Autodesk Inventor part; units mm, degrees
ref_plane "YZ Plane" through (0, 0, 0) normal (1, 0, 0) x (0, 1, 0)
ref_plane "XZ Plane" through (0, 0, 0) normal (0, 1, 0) x (-1, 0, 0)
ref_plane "XY Plane" through (0, 0, 0) normal (0, 0, 1) x (1, 0, 0)
ref_plane "Work Plane5" through (0, 0, 10) normal (0, 0, 1) x (1, 0, 0)
sketch "Sketch1" plane through (0, 0, 10) normal (0, 0, 1) x (1, 0, 0)
  line L0 (-4.0299, -0.3538) -> (-2.2322, 1.4439) construction
  arc A0 (-1.4439, 2.2322) -> (-2.2322, 1.4439) centre (-0.9299, 0.9299) ccw construction
  line L1 (-1.4439, 2.2322) -> (0.3538, 4.0299) construction
  line L2 (-37.8299, 42.8299) -> (-37.8299, 37.8299) construction
  line L3 (-37.8299, 37.8299) -> (-42.9208, 37.8299) construction
  line L4 (-37.8299, 42.2137) -> (-37.8299, 45.8299) construction
  line L5 (-37.8299, 45.8299) -> (-4.0299, 45.8299) construction
  line L6 (-4.0299, 45.8299) -> (-4.0299, 42.2137) construction
  line L7 (-4.0299, 4.0299) -> (0.3538, 4.0299)
  circle A1 centre (-20.9299, 20.9299) radius 17.5
  line L8 (-20.9299, 58.9723) -> (17.1124, 20.9299) construction
  line L9 (17.1124, 20.9299) -> (-20.9299, -17.1124) construction
  line L10 (-20.9299, -17.1124) -> (-58.9723, 20.9299) construction
  line L11 (-58.9723, 20.9299) -> (-20.9299, 58.9723) construction
  line L12 (-20.9299, 58.9723) -> (-20.9299, -17.1124) construction
  line L13 (17.1124, 20.9299) -> (-58.9723, 20.9299) construction
  line L14 (-20.9299, 58.9723) -> (32.8701, 58.9723) construction
  line L15 (-43.4299, 43.4299) -> (1.5701, 43.4299) construction
  line L16 (1.5701, 43.4299) -> (1.5701, -1.5701) construction
  line L17 (1.5701, -1.5701) -> (-43.4299, -1.5701) construction
  line L18 (-43.4299, -1.5701) -> (-43.4299, 43.4299) construction
  line L19 (-43.4299, 43.4299) -> (1.5701, -1.5701) construction
  line L20 (1.5701, 43.4299) -> (-43.4299, -1.5701) construction
  line L21 (-43.4299, 5.3876) -> (-43.4299, 36.4723)
  line L22 (-43.4299, 36.4723) -> (-36.4723, 43.4299)
  line L23 (-36.4723, 43.4299) -> (-5.3876, 43.4299)
  line L24 (-5.3876, 43.4299) -> (1.5701, 36.4723)
  line L25 (1.5701, 36.4723) -> (1.5701, 5.3876)
  line L26 (1.5701, 5.3876) -> (-5.3876, -1.5701)
  line L27 (-5.3876, -1.5701) -> (-36.4723, -1.5701)
  line L28 (-36.4723, -1.5701) -> (-43.4299, 5.3876)
  line L29 (-4.0299, 42.2137) -> (-37.8299, 42.2137)
  line L30 (-4.0299, -0.3538) -> (-4.0299, 4.0299)
  circle A2 centre (-20.9299, 20.9299) radius 1.5
  line L31 (-10.9299, 10.9299) -> (-30.9299, 10.9299) construction
  line L32 (-30.9299, 10.9299) -> (-30.9299, 30.9299) construction
  line L33 (-30.9299, 30.9299) -> (-10.9299, 30.9299) construction
  line L34 (-10.9299, 30.9299) -> (-10.9299, 10.9299) construction
  line L35 (-10.9299, 10.9299) -> (-30.9299, 30.9299) construction
  line L36 (-30.9299, 10.9299) -> (-10.9299, 30.9299) construction
  circle A3 centre (-30.9299, 30.9299) radius 1.4
  circle A4 centre (-30.9299, 10.9299) radius 1.4
  circle A5 centre (-10.9299, 10.9299) radius 1.4
  line L37 (-45.8299, 37.8299) -> (-42.0723, 37.8299) construction
  line L38 (-42.1723, 37.7299) -> (-45.8299, 37.7299)
  line L39 (-45.8299, 37.7299) -> (-45.8299, 4.1299)
  line L40 (-45.8299, 4.1299) -> (-42.1723, 4.1299)
  line L41 (-42.1723, 4.1299) -> (-42.1723, 37.7299)
  line L42 (-45.8299, 4.0299) -> (-42.0723, 4.0299) construction
  line L43 (-45.8299, 37.8299) -> (-42.0723, 37.8299)
  line L44 (-37.7299, 45.8299) -> (-4.1299, 45.8299)
  line L45 (-4.1299, 45.8299) -> (-4.1299, 42.1723)
  line L46 (-4.1299, 42.1723) -> (-37.7299, 42.1723)
  line L47 (-37.7299, 42.1723) -> (-37.7299, 45.8299)
  line L48 (0.4701, 37.8299) -> (0.4701, 4.0299) construction
  line L49 (0.4701, 4.0299) -> (3.9701, 4.0299) construction
  line L50 (3.9701, 37.8299) -> (3.9701, 4.0299) construction
  line L51 (0.4701, 37.8299) -> (3.9701, 37.8299) construction
  line L52 (-45.8299, -3.9701) -> (-4.0299, -3.9701) construction
  line L53 (0.3124, 37.7299) -> (3.9701, 37.7299)
  line L54 (3.9701, 37.7299) -> (3.9701, 4.1299)
  line L55 (3.9701, 4.1299) -> (0.3124, 4.1299)
  line L56 (0.3124, 4.1299) -> (0.3124, 37.7299)
  line L57 (-4.1713, -0.3538) -> (-37.7299, -0.3538)
  line L58 (-37.7299, -0.3538) -> (-37.7299, -3.9701)
  line L59 (-37.7299, -3.9701) -> (-4.1713, -3.9701)
  line L60 (-4.1713, -3.9701) -> (-4.1713, -0.3538)
  point P0 (-37.8299, 4.0299)
  dimension "d18" = 53.8
  dimension "d19" = 45
  dimension "d20" = 53.8
  dimension "d21" = 45
  dimension "d22" = 45
  dimension "d30" = 20
  dimension "d31" = 20
  dimension "d32" = 2.8
  dimension "d33" = 2.8
  dimension "d34" = 2.8
  dimension "d35" = 3
  dimension "d36" = 0.1
  dimension "d37" = 0.1
  dimension "d38" = 0.1
  dimension "d39" = 0.1
extrude "Extrusion1" add sketch "Sketch1" along normal blind 15 contours L30 L26 L57 L28 L41 L22 L46 L24 L56 L7 | L7 L26 L30 | L56 L24 L25 L26 | L26 L25 L24 L53 L54 L55 | L60 L59 L58 L57 L28 L27 L26 | L26 L27 L28 L57 | L46 L22 L29 L24 | L24 L29 L45 | L40 L39 L38 L22 L21 L28 | L28 L21 L22 L41 | L29 L22 L23 L24 | L24 L23 L22 L29 L47 L44 L45 | L47 L29 L22 | A1 | A2 | A3 | A4 | A5
sketch "Skizze4" plane through (0, 0, 25) normal (0, 0, 1) x (1, 0, 0)
  line L0 (-37.7299, 42.1723) -> (-42.1723, 37.7299)
  line L1 (-42.1723, 37.7299) -> (-45.8299, 37.7299)
  line L2 (-45.8299, 37.7299) -> (-45.8299, 4.1299) construction
  line L3 (-45.8299, 4.1299) -> (-42.1723, 4.1299)
  line L4 (-42.1723, 4.1299) -> (-37.6885, -0.3538)
  line L5 (-37.6885, -0.3538) -> (-37.7299, -0.3538)
  line L6 (-37.7299, -0.3538) -> (-37.7299, -3.9701)
  line L7 (-37.7299, -3.9701) -> (-4.1713, -3.9701) construction
  line L8 (-4.1713, -3.9701) -> (-4.1713, -0.3538)
  line L9 (-4.1713, -0.3538) -> (0.3124, 4.1299)
  line L10 (0.3124, 4.1299) -> (3.9701, 4.1299)
  line L11 (3.9701, 4.1299) -> (3.9701, 37.7299) construction
  line L12 (3.9701, 37.7299) -> (0.3124, 37.7299)
  line L13 (0.3124, 37.7299) -> (-4.1299, 42.1723)
  line L14 (-4.1299, 42.1723) -> (-4.1299, 45.8299)
  line L15 (-4.1299, 45.8299) -> (-37.7299, 45.8299) construction
  line L16 (-37.7299, 45.8299) -> (-37.7299, 42.1723)
  line L17 (-37.9299, 46.0299) -> (-3.9299, 46.0299) construction
  line L18 (-3.9299, 46.0299) -> (-3.9299, 42.2551)
  line L19 (-3.9299, 42.2551) -> (0.3953, 37.9299)
  line L20 (0.3953, 37.9299) -> (4.1701, 37.9299)
  line L21 (4.1701, 37.9299) -> (4.1701, 3.9299) construction
  line L22 (4.1701, 3.9299) -> (0.3953, 3.9299)
  line L23 (0.3953, 3.9299) -> (-3.9713, -0.4367)
  line L24 (-3.9713, -0.4367) -> (-3.9713, -4.1701)
  line L25 (-3.9713, -4.1701) -> (-37.9299, -4.1701) construction
  line L26 (-37.9299, -4.1701) -> (-37.9299, -0.3953)
  line L27 (-37.9299, -0.3953) -> (-42.2551, 3.9299)
  line L28 (-42.2551, 3.9299) -> (-46.0299, 3.9299)
  line L29 (-46.0299, 3.9299) -> (-46.0299, 37.9299) construction
  line L30 (-46.0299, 37.9299) -> (-42.2551, 37.9299)
  line L31 (-42.2551, 37.9299) -> (-37.9299, 42.2551)
  line L32 (-37.9299, 42.2551) -> (-37.9299, 46.0299)
  line L33 (-45.8299, 37.7299) -> (-45.8299, 37.9299)
  line L34 (-4.1299, 45.8299) -> (-37.7299, 45.8299)
  line L35 (-37.7299, 45.8299) -> (-37.9299, 45.8299)
  line L36 (-4.1299, 45.8299) -> (-3.9299, 45.8299)
  line L37 (3.9701, 37.7299) -> (3.9701, 37.9299)
  line L38 (3.9701, 4.1299) -> (3.9701, 37.7299)
  line L39 (3.9701, 4.1299) -> (3.9701, 3.9299)
  line L40 (-4.1713, -3.9701) -> (-3.9713, -3.9701)
  line L41 (-37.7299, -3.9701) -> (-37.9299, -3.9701)
  line L42 (-45.8299, 4.1299) -> (-45.8299, 3.9299)
  point P0 (0, 0)
  dimension "d40" = 0.2
extrude "IM_offset" add sketch "Skizze4" against normal up to surface (15 mm away)
sketch "Sketch29" plane through (0, 0, 10) normal (0, 0, -1) x (-1, 0, 0)
  arc A0 (6.7299, 9.4299) -> (9.4299, 6.7299) centre (9.4299, 9.4299) ccw
  line L0 (9.4299, 6.7299) -> (32.4299, 6.7299)
  arc A1 (32.4299, 6.7299) -> (35.1299, 9.4299) centre (32.4299, 9.4299) ccw
  line L1 (35.1299, 9.4299) -> (35.1299, 32.4299)
  arc A2 (35.1299, 32.4299) -> (32.4299, 35.1299) centre (32.4299, 32.4299) ccw
  line L2 (32.4299, 35.1299) -> (9.4299, 35.1299)
  arc A3 (9.4299, 35.1299) -> (6.7299, 32.4299) centre (9.4299, 32.4299) ccw
  line L3 (6.7299, 32.4299) -> (6.7299, 9.4299)
  line L4 (36.9299, 4.9299) -> (4.9299, 4.9299)
  line L5 (4.9299, 4.9299) -> (4.9299, 36.9299)
  line L6 (4.9299, 36.9299) -> (36.9299, 36.9299)
  line L7 (36.9299, 36.9299) -> (36.9299, 4.9299)
  line L8 (36.9299, 4.9299) -> (4.9299, 36.9299) construction
  line L9 (4.9299, 4.9299) -> (36.9299, 36.9299) construction
  point P0 (0, 0)
  point P1 (20.9299, 20.9299)
  dimension "d187" = 32
  dimension "d188" = 32
extrude "Extrusion23" cut sketch "Sketch29" against normal through all contours L3 A3 L2 A2 L1 A1 L0 A0 | L4 L5 L6 L7
sketch "Sketch30" plane through (-45.8299, 0, 10) normal (-1, 0, 0) x (0, 0, 1)
  line L0 (35.0799, 45.8299) -> (6.8799, 45.8299)
  line L1 (0, 3.9299) -> (0, 37.9299)
  line L2 (15, 3.9299) -> (0, 3.9299)
  line L3 (15, 37.9299) -> (15, 3.9299)
  line L4 (15, 37.9299) -> (0, 37.9299)
  circle A0 centre (7.5, 20.9299) radius 1.7201
  point P0 (-10, 0)
ref_plane "Arbeitsebene7" through (-20.9299, 3.9299, 10) normal (-1, 0, 0) x (0, 0, 1)
ref_plane "Arbeitsebene8" through (-37.9299, 20.9299, 10) normal (0, 1, 0) x (1, 0, 0)
ref_plane "Arbeitsebene9" through (-20.9299, 3.9299, 10) normal (-1, 0, 0) x (0, 0, 1)
ref_plane "Arbeitsebene10" through (-37.9299, 20.9299, 10) normal (0, -1, 0) x (1, 0, 0)
hole "Bohrung2" at (-45.8299, 20.9299, 17.5) direction (1, 0, 0) diameter 2.8 end through all counterbore diameter 6 counterbore depth 4
pattern_circular "Runde Anordnung2" count 4 over 360 about axis through (-20.9299, 20.9299, 10) along (0, 0, 1) of "Bohrung2"
ref_plane "Arbeitsebene11" through (-20.9299, 3.9299, 10) normal (1, 0, 0) x (0, 0, -1)
ref_plane "Arbeitsebene12" through (-37.9299, 20.9299, 10) normal (0, 1, 0) x (1, 0, 0)
properties part number "30_Cube_Z_Focus_MGN_NEMA_Motorsupport_centered"
CAD build for the part. Positions are in the model's coordinates, mm. A direction names the side the tool comes from. Round coordinates to 2 decimals unless told otherwise and drop trailing zeros. Order: outer loops, then holes, each group sorted by start corner. A loop starts at its lowest first (then second) coordinate and runs counter-clockwise, first axis right, second up. Notation, with made-up numbers: (2.25, 9) -> (21.25, 9) arc R16 cw to (21.25, 37) -> close; hole circle Ø10 at (-35.75, 43). An arc over 180 degrees is marked (long way). One line per question, with ' | ' between items.
Q1. Slice it at C-C (x = -3). Write the cut outline in (y, z), then the cut area to 3 significant figures.
Completed:
outline: (0.53, 10) -> (41.33, 10) -> (41.33, 25) -> (0.53, 25) -> close; hole circle Ø2.8 at (20.93, 17.5) | area: 606 mm^2
Q2. Which spindle directions (+Z, -Z, +X, -X, +Y, -Y) get a long thin tool onto all of the face, cutting with end or side? Do faces 4 (the flat face through (2, 3.93, 18)), 5 (the cylindrical face through (-43.802, 22.755, 15.119)), 6 (the flat face through (-37.93, -2, 18)). Say none if no direction does.
Completed:
face 4: +Z, -Z, +X, -Y | face 5: -X | face 6: +Z, -Z, -X, -Y
Q3. Two-plate mould, pull along Z, no slides. Class faces 1 (the flat face through (-22, 0.03, 19)), 2 (the flat face through (-4.93, 20.7, 15.7)), 3 (the flat face through (-21, 38, 10)): released by +Z, released by -Z, zero draft, split by the parting line, or undercut.
Completed:
face 1: undercut | face 2: zero draft | face 3: released by -Z
Q4. Probe probe 1 along Y at (x, z) = (-31.5, 19); probe 2 along X at (y, z) = (-2.9, 17.5); probe 3 along Y at (x, z) = (-43.85, 17.5). List the from-to ranges inside material, lowest first.
Completed:
probe 1: y = -3.97 to 4.93, 36.93 to 45.83 | probe 2: x = -37.93 to -23.93, -17.93 to -3.97 | probe 3: y = 3.93 to 17.93, 23.93 to 37.93
Q5. Slice it at B-B (x = -11.5). Write the cut outline in (y, z).
Completed:
outline: (-3.97, 10) -> (4.93, 10) -> (4.93, 25) -> (-3.97, 25) -> close; (36.93, 10) -> (45.83, 10) -> (45.83, 25) -> (36.93, 25) -> close
Q6. Slice it at D-D (z = 17.5). Give the number of separate pieces and of enclosed holes in the cut face, then the cut area to 3 significant figures.
Completed:
separate pieces: 4 | enclosed holes: 0 | area: 1,090 mm^2
Q7. Slice it at A-A (y = 33.5). Write the cut outline in (x, z), then the cut area to 3 significant figures.
Completed:
outline: (-45.83, 10) -> (-36.93, 10) -> (-36.93, 25) -> (-45.83, 25) -> close; (-4.93, 10) -> (3.97, 10) -> (3.97, 25) -> (-4.93, 25) -> close | area: 267 mm^2
Q8. Drop flat-ended pins along their axis: pin 1 (2 mm diameter, centred on y = 20.93, z = 17.5, fed in from +X); pin 2 (1.1 mm diameter, centred on y = -2, z = 18.5, fed in from -X); pin 3 (3 mm diameter, centred on y = 43.5, z = 15, fed in from -X) (3 decimals); pin 4 (3.5 mm diameter, centred on x = -20.93, z = 17.5, fed in from +Y). Give the stop position or say it passes through.
Completed:
pin 1: passes through | pin 2: stops at x = -37.93 | pin 3: stops at x = -38.185 | pin 4: stops at y = 41.83
